Here's how the part is built. I have some questions about the finished solid (model axes, mm). A direction names the side the tool comes from. Round coordinates to 2 decimals unless told otherwise and drop trailing zeros. Order: outer loops, then holes, each group sorted by start corner. A loop starts at its lowest first (then second) coordinate and runs counter-clockwise, first axis right, second up.
```python
from build123d import *

# Parameters (mm, degrees)
SM_BASE_FLANGE_1_DEPTH = 113
CUT_EXTRUDE_1_DEPTH    = 10
CUT_EXTRUDE_2_DEPTH    = 10
CHAMFER_1_SIZE         = 5
SKETCH_8_W             = 195
SKETCH_8_H             = 40
CUT_EXTRUDE_3_DEPTH    = 10


# Sheet-metal steps are written as plain solids
with BuildPart() as part:
    # Sketch 1 → 基体-法兰1 (new, symmetric)
    with BuildSketch(Plane.XY):
        with BuildLine():
            Line((0, 100), (0, 3.1))
            ThreePointArc((0, 3.1), (-0.907968978, 0.907968978), (-3.1, 0))
            Line((-3.1, 0), (-48, 0))
            Line((-48, 0), (-48, 3))
            Line((-48, 3), (-3.1, 3))
            ThreePointArc((-3.1, 3), (-3.029289322, 3.029289322), (-3, 3.1))
            Line((-3, 3.1), (-3, 100))
            Line((-3, 100), (0, 100))
        make_face()
    extrude(amount=SM_BASE_FLANGE_1_DEPTH, both=True)

    # 草图6 → 切除-拉伸1 (cut)
    with BuildSketch(Plane.ZY.offset(3)):
        with BuildLine():
            Line((-102.4, 92), (-102.4, 58))
            ThreePointArc((-102.4, 58), (-105, 55.4), (-107.6, 58))
            Line((-107.6, 58), (-107.6, 92))
            ThreePointArc((-107.6, 92), (-105, 94.6), (-102.4, 92))
        make_face()
        with BuildLine():
            Line((107.6, 92), (107.6, 58))
            ThreePointArc((107.6, 58), (105, 55.4), (102.4, 58))
            Line((102.4, 58), (102.4, 92))
            ThreePointArc((102.4, 92), (105, 94.6), (107.6, 92))
        make_face()
    extrude(amount=-CUT_EXTRUDE_1_DEPTH, mode=Mode.SUBTRACT)

    # 草图7 → 切除-拉伸2 (cut)
    with BuildSketch(Plane(origin=(0, 3, 0), x_dir=(1, 0, 0), z_dir=(0, 1, 0))):
        with BuildLine():
            Line((-35, 102.6), (-15, 102.6))
            ThreePointArc((-15, 102.6), (-12.4, 100), (-15, 97.4))
            Line((-15, 97.4), (-35, 97.4))
            ThreePointArc((-35, 97.4), (-37.6, 100), (-35, 102.6))
        make_face()
        with BuildLine():
            Line((-35, 2.6), (-15, 2.6))
            ThreePointArc((-15, 2.6), (-12.4, 0), (-15, -2.6))
            Line((-15, -2.6), (-35, -2.6))
            ThreePointArc((-35, -2.6), (-37.6, 0), (-35, 2.6))
        make_face()
        with BuildLine():
            Line((-35, -97.4), (-15, -97.4))
            ThreePointArc((-15, -97.4), (-12.4, -100), (-15, -102.6))
            Line((-15, -102.6), (-35, -102.6))
            ThreePointArc((-35, -102.6), (-37.6, -100), (-35, -97.4))
        make_face()
    extrude(amount=-CUT_EXTRUDE_2_DEPTH, mode=Mode.SUBTRACT)

    # 倒角1
    chamfer_1_edges = [part.edges().sort_by_distance(p)[0] for p in [
        (-1.5, 100, 113),
        (-48, 1.5, 113),
        (-1.5, 100, -113),
        (-48, 1.5, -113),
    ]]
    chamfer(chamfer_1_edges, length=CHAMFER_1_SIZE)

    # 草图8 → 切除-拉伸3 (cut)
    with BuildSketch(Plane.ZY.offset(3)):
        with Locations((0, 100)):
            Rectangle(SKETCH_8_W, SKETCH_8_H)
    extrude(amount=-CUT_EXTRUDE_3_DEPTH, mode=Mode.SUBTRACT)


solid = part.part
```
1. If we section it at A-A, the plane z = 105: Write out the boundary of the cut face in (x, y).
Evaluation:
outline: (-48, 0) - (-3.1, 0) arc R3.1 ccw to (0, 3.1) - (0, 55.4) - (-3, 55.4) - (-3, 3.1) arc R0.1 cw to (-3.1, 3) - (-48, 3) - close; (-3, 94.6) - (0, 94.6) - (0, 100) - (-3, 100) - close
2. If we section it at D-D, the plane y = 52.5: Write out the boundary of the cut face in (x, z).
Evaluation:
outline: (-3, -113) - (0, -113) - (0, 113) - (-3, 113) - close
3. On a 3-axis mill with a long thin cutter (end or side, diameter ignored), from which of +Z, -Z, +X, -X, +Y, -Y can I reach the whole of each face in a straight line? I mean faces 1 (the flat face through (-2, 97, -111)), 2 (the flat face through (-11, 3, 2)). Say none if no direction works.
Evaluation:
face 1: -Z, +X, -X, +Y
face 2: +Z, -Z, -X, +Y
4. I need wall thicknesses on probe 1 along Y at (x, z) = (-11, -19); probe 2 along X at (y, z) = (65, 49). Which ranges of each line are inside material? Lowest first, please.
Evaluation:
probe 1: y = 0 to 3
probe 2: x = -3 to 0
5. I'm going to push flat-ended pins straight in: P1, Ø12, axis at x = -34.5, z = 58, coming from the +Y side; P2, Ø0.9, axis at x = -1.5, z = -46, coming from the +Y side; P3, Ø6, axis at y = 17.5, z = 13.5, coming from the -X side. Where does each tip first touch, or does it pass through?
Evaluation:
P1: stops at y = 3
P2: stops at y = 80
P3: stops at x = -3
6. If we section it at B-B, the plane x = -20.5: Write out the boundary of the cut face in (y, z), and give its area (3 significant figures).
Evaluation:
outline: (0, -113) - (3, -113) - (3, -102.6) - (0, -102.6) - close; (0, -97.4) - (3, -97.4) - (3, -2.6) - (0, -2.6) - close; (0, 2.6) - (3, 2.6) - (3, 97.4) - (0, 97.4) - close; (0, 102.6) - (3, 102.6) - (3, 113) - (0, 113) - close
area: 631 mm2
7. If we section it at C-C, the plane z = -17: Write out the boundary of the cut face in (x, y).
Evaluation:
outline: (-48, 0) - (-3.1, 0) arc R3.1 ccw to (0, 3.1) - (0, 80) - (-3, 80) - (-3, 3.1) arc R0.1 cw to (-3.1, 3) - (-48, 3) - close
